Check sheet for the modelled part. Datum: model origin and axes. Units: mm. Face numbers are marked on the shaded views. A direction names the side the tool comes from. Give positions to 0.01 mm unless a question says otherwise; leave off trailing zeros. Loops run counter-clockwise (first coordinate to the right, second up) from the corner with the lowest first, then second, coordinate; pieces in that order, holes last. Notation, with made-up numbers: (13, 84) -> (40, 84) arc R24 cw to (40, 116) -> close; hole circle Ø1 at (21, -32). An arc over 180 degrees is marked (long way). Write each question's results on one line, items separated by ' | '. Start each with the question number.
1. Cross-section at B-B on z = 14.5. Record the boundary of the cut face in (x, y), and give its area (3 significant figures).
2. Material ranges on L1, parallel to Y at x = 8.5, z = 15.5; L2, parallel to Y at x = -37.95, z = 12.7; L3, parallel to X at y = 9, z = 7.75, recorded low to high. Write a range as from..to.
3. Mould release check, pull along Y, two halves, no side actions. Record for the marked faces 1, 2, 3 and 4: +Y half, -Y half, draft (parallel to the pull), parting line (faces both ways), or undercut.
4. Tool access check on the marked faces 5 and 6. Record the directions out of +Z, -Z, +X, -X, +Y, -Y that give a thin tool (end or side, any length) a straight path to the whole face; none if there is none.
5. Cross-section at A-A on y = 11. Record the boundary of the cut face in (x, z).
6. Gauge pin test, flat ends, axial feed: pin 1 Ø6 at (x, z) = (-17, 9) entering from -Y; pin 2 Ø1.5 at (y, z) = (-15.5, 12.5) entering from -X. Record the tip position at first contact, or that the pin passes through.
7. Cross-section at C-C on x = 4.5. Record the boundary of the cut face in (y, z).
from build123d import *

# Parameters (mm, degrees)
F0_W      = 83.82
F0_H      = 50.8
F1_DEPTH  = 3.81
F2_W      = 83.82
F2_H      = 50.8
F2_W_2    = 76.2
F2_H_2    = 43.18
F3_DEPTH  = 21.59
F5_DEPTH  = 5.08
F7_DEPTH  = 25.4
F8_SIZE2  = 1.27
F8_SIZE   = 1.27
F9_W      = 8.128
F9_H      = 4.318
F10_DEPTH = 25.4


with BuildPart() as f1:
    # F0 (on Top) → F1 (new body)
    with BuildSketch(Plane.XY):
        with Locations((0.872821, -2.059813)):
            Rectangle(F0_W, F0_H)
    extrude(amount=F1_DEPTH)

    # F2 (on face) → F3 (join)
    with BuildSketch(Plane.XY.offset(3.81)):
        with Locations((0.872821, -2.059813)):
            Rectangle(F2_W, F2_H)
        with Locations((1.016111, -1.792254)):
            Rectangle(F2_W_2, F2_H_2, mode=Mode.SUBTRACT)
    extrude(amount=F3_DEPTH)

    # F4 (on face) → F5 (cut)
    with BuildSketch(Plane.XZ.offset(27.459813)):
        with BuildLine():
            ThreePointArc((-23.892179, 12.7), (-15.637179, 4.445), (-7.382179, 12.7))
            ThreePointArc((-7.382179, 12.7), (-9.800013, 18.537166), (-15.637179, 20.955))
            Line((-15.637179, 20.955), (-15.637179, 12.7))
            Line((-15.637179, 12.7), (-23.892179, 12.7))
        make_face()
        with BuildLine():
            Line((-15.637179, 12.7), (-15.637179, 20.955))
            ThreePointArc((-15.637179, 20.955), (-21.474346, 18.537166), (-23.892179, 12.7))
            Line((-23.892179, 12.7), (-15.637179, 12.7))
        make_face()
    extrude(amount=-F5_DEPTH, mode=Mode.SUBTRACT)

    # F6 (on face) → F7 (cut)
    with BuildSketch(Plane(origin=(-41.037179, 0, 0), x_dir=(0, -1, 0), z_dir=(-1, 0, 0))):
        with BuildLine():
            Line((14.759813, 12.7), (19.204813, 12.7))
            ThreePointArc((19.204813, 12.7), (17.902903, 15.84309), (14.759813, 17.145))
            Line((14.759813, 17.145), (14.759813, 12.7))
        make_face()
        with BuildLine():
            ThreePointArc((14.759813, 17.145), (11.616724, 9.55691), (19.204813, 12.7))
            Line((19.204813, 12.7), (14.759813, 12.7))
            Line((14.759813, 12.7), (14.759813, 17.145))
        make_face()
    extrude(amount=-F7_DEPTH, mode=Mode.SUBTRACT)

    # F8
    f8_edges = [f1.edges().sort_by_distance(p)[0] for p in [
        (1.016111, 19.797746, 25.4),
        (-37.083889, -1.792254, 25.4),
        (1.016111, -23.382254, 25.4),
        (39.116111, -1.792254, 25.4),
    ]]
    chamfer(f8_edges, length=F8_SIZE, length2=F8_SIZE2)

    # F9 (on face) → F10 (cut)
    with BuildSketch(Plane.YZ.offset(42.782821)):
        with Locations((-13.235813, 8.509)):
            Rectangle(F9_W, F9_H)
    extrude(amount=-F10_DEPTH, mode=Mode.SUBTRACT)


solid = f1.part
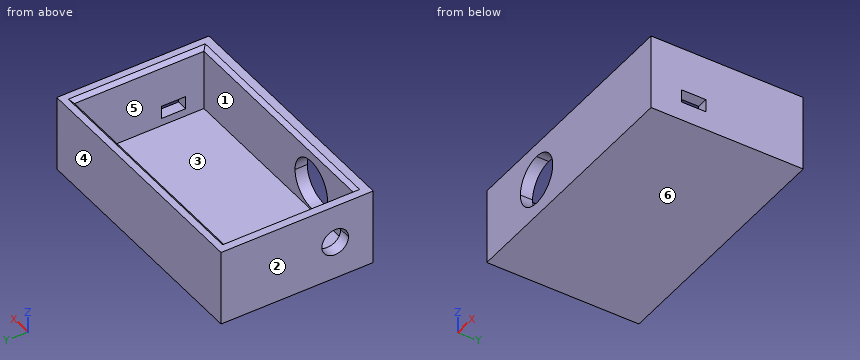
Geometry says:
1) outline: (-41.04, -27.46) -> (-23.69, -27.46) -> (-23.69, -23.38) -> (-37.08, -23.38) -> (-37.08, -18.82) -> (-41.04, -18.82) -> close; (-41.04, -10.7) -> (-37.08, -10.7) -> (-37.08, 19.8) -> (39.12, 19.8) -> (39.12, -23.38) -> (-7.58, -23.38) -> (-7.58, -27.46) -> (42.78, -27.46) -> (42.78, 23.34) -> (-41.04, 23.34) -> close | area: 870 mm^2
2) L1: -27.46..-23.38, 19.8..23.34 | L2: -27.46..-19.2, -10.31..23.34 | L3: -41.04..-37.08, 39.12..42.78
3) face 1: undercut | face 2: draft | face 3: undercut | face 4: +Y half
4) face 5: +Z | face 6: -Z, +X, -X, +Y, -Y
5) outline: (-41.04, 0) -> (42.78, 0) -> (42.78, 25.4) -> (40.39, 25.4) -> (39.12, 24.13) -> (39.12, 3.81) -> (-37.08, 3.81) -> (-37.08, 24.13) -> (-38.35, 25.4) -> (-41.04, 25.4) -> close
6) pin 1: y = 19.8 | pin 2: x = 39.12
7) outline: (-27.46, 0) -> (23.34, 0) -> (23.34, 25.4) -> (21.07, 25.4) -> (19.8, 24.13) -> (19.8, 3.81) -> (-23.38, 3.81) -> (-23.38, 24.13) -> (-24.65, 25.4) -> (-27.46, 25.4) -> close
